CAD build for the part. Positions are in the model's coordinates, mm. Face numbers are marked on the shaded views. A direction names the side the tool comes from. Give positions to 0.01 mm unless a question says otherwise; leave off trailing zeros. Order: outer loops, then holes, each group sorted by start corner. A loop starts at its lowest first (then second) coordinate and runs counter-clockwise, first axis right, second up.
Item 1: Band-saw the part on B-B on y = 0. Give the cut face in (x, z), plus the area to 3 significant figures.
Item 2: Flat gauge pins, fed straight in: P1, Ø1, axis at x = -4, z = 1.5, coming from the +Y side; P2, Ø1, axis at x = 1.5, y = 0, coming from the +Z side; P3, Ø1, axis at x = 4.5, z = 2, coming from the -Y side. Where does each tip first touch, or does it go through?
Item 3: Two-plate mould, pull along X, no slides. Class the marked faces 1, 2 and 3: released by +X, released by -X, zero draft, split by the parting line, or undercut.
Item 4: Which spindle directions (+Z, -Z, +X, -X, +Y, -Y) get a long thin tool onto all of the face, cutting with end or side? Do the marked faces 4 and 5. Say none if no direction does.
Item 5: Band-saw the part on A-A on x = 0. Give the cut face in (y, z), plus the area to 3 significant figures.
Item 6: Band-saw the part on C-C on z = 1.85. Give the cut face in (x, y), plus the area to 3 significant figures.
Item 7: Wall check: L1, parallel to Y at x = 0, z = 1.8; L2, parallel to X at y = 1.75, z = 1.05; L3, parallel to X at y = -2.5, z = 1.6. Give the ranges that are in metal, low to high.
```python
from build123d import *

# Parameters (mm, degrees)
F2_W     = 4.224532
F2_H     = 1.6
F3_DEPTH = 4


with BuildPart() as f1:
    # F0 (on Front) → F1 (revolve)
    with BuildSketch(Plane.XZ):
        with BuildLine():
            ThreePointArc((3.5, 0.3), (3.587868, 0.087868), (3.8, 0))
            Line((3.8, 0), (5.2, 0))
            ThreePointArc((5.2, 0), (5.412132, 0.087868), (5.5, 0.3))
            Line((5.5, 0.3), (5.5, 3))
            Line((5.5, 3), (3.5, 3))
            Line((3.5, 3), (3.5, 0.3))
        make_face()
    revolve(axis=Axis((0, 0, 3.851013), (0, 0, 1)))

    # F2 (on Top) → F3 (cut)
    with BuildSketch(Plane.XY):
        with Locations((4.5, 0)):
            Rectangle(F2_W, F2_H)
    extrude(amount=F3_DEPTH, mode=Mode.SUBTRACT)


solid = f1.part
```
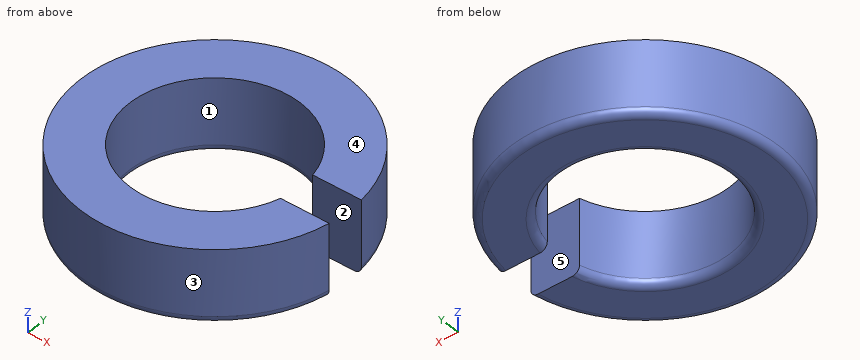
The answers:
1. outline: (-5.5, 0.3) arc R0.3 ccw to (-5.2, 0) - (-3.8, 0) arc R0.3 ccw to (-3.5, 0.3) - (-3.5, 3) - (-5.5, 3) - close
1. area: 5.96 mm2
2. P1: stops at y = 4.24
2. P2: passes through
2. P3: stops at y = -3.77
3. face 1: undercut
3. face 2: zero draft
3. face 3: split by the parting line
4. face 4: +Z, +X, -X, +Y, -Y
4. face 5: +Z, -Z, +X
5. outline: (-5.5, 0.3) arc R0.3 ccw to (-5.2, 0) - (-3.8, 0) arc R0.3 ccw to (-3.5, 0.3) - (-3.5, 3) - (-5.5, 3) - close; (3.5, 0.3) arc R0.3 ccw to (3.8, 0) - (5.2, 0) arc R0.3 ccw to (5.5, 0.3) - (5.5, 3) - (3.5, 3) - close
5. area: 11.9 mm2
6. outline: (3.41, -0.8) arc R3.5 cw (long way) to (3.41, 0.8) - (5.44, 0.8) arc R5.5 ccw (long way) to (5.44, -0.8) - close
6. area: 53.3 mm2
7. L1: y = -5.5 to -3.5, 3.5 to 5.5
7. L2: x = -5.21 to -3.03, 3.03 to 5.21
7. L3: x = -4.9 to -2.45, 2.45 to 4.9
